Build history of the part. All positions in model axes, mm. Round coordinates to 2 decimals unless told otherwise and drop trailing zeros. Loops run counter-clockwise (first coordinate to the right, second up) from the corner with the lowest first, then second, coordinate; pieces in that order, holes last.
from build123d import *

# Parameters (mm, degrees)
F0_W     = 50.8
F0_H     = 101.6
F0_R     = 7.62
F1_DEPTH = 25.4
F2_R     = 5.08
F3_R     = 3.752901
F4_DEPTH = 25.4


with BuildPart() as f1:
    # F0 (on Front) → F1 (new body)
    with BuildSketch(Plane.XZ):
        Rectangle(F0_W, F0_H)
        with Locations((0, -26.934734)):
            Circle(F0_R, mode=Mode.SUBTRACT)
        with Locations((0, 26.934734)):
            Circle(F0_R, mode=Mode.SUBTRACT)
    extrude(amount=F1_DEPTH)

    # F2
    f2_edges = [f1.edges().sort_by_distance(p)[0] for p in [
        (25.4, -12.7, -50.8),
        (25.4, -12.7, 50.8),
        (-25.4, -12.7, 50.8),
        (-25.4, -12.7, -50.8),
    ]]
    fillet(f2_edges, radius=F2_R)

    # F3 (on face) → F4 (cut)
    with BuildSketch(Plane(origin=(0, 0, 0), x_dir=(-1, 0, 0), z_dir=(0, 1, 0))):
        with Locations((-15.947323, 40.916275)):
            Circle(F3_R)
        with Locations((15.947323, 40.916275)):
            Circle(F3_R)
        with Locations((15.947323, -40.916275)):
            Circle(F3_R)
        with Locations((-15.947323, -40.916275)):
            Circle(F3_R)
    extrude(amount=-F4_DEPTH, mode=Mode.SUBTRACT)


solid = f1.part
(1) Probe line 1 (Z direction, x = 0, y = -19.5); line 2 (X direction, y = -15, z = -40.5); line 3 (Z direction, x = 16, y = -14.5). List the from-to ranges inside material, lowest first.
Responses:
line 1: z = -50.8 to -34.55, -19.31 to 19.31, 34.55 to 50.8
line 2: x = -25.4 to -19.68, -12.22 to 12.22, 19.68 to 25.4
line 3: z = -50.8 to -44.67, -37.16 to 37.16, 44.67 to 50.8
(2) Pin check, flat tip, straight feed: P1, Ø6, axis at x = 15.95, z = 40.92, coming from the +Y side. Stop position of the tip, or through.
Responses:
P1: passes through
(3) Slice it at C-C on y = -12. List the corners of the cut face in (x, z), plus the area to 3 significant figures.
Responses:
outline: (-25.4, -45.72) arc R5.08 ccw to (-20.32, -50.8) - (20.32, -50.8) arc R5.08 ccw to (25.4, -45.72) - (25.4, 45.72) arc R5.08 ccw to (20.32, 50.8) - (-20.32, 50.8) arc R5.08 ccw to (-25.4, 45.72) - close; hole circle Ø7.51 at (-15.95, -40.92); hole circle Ø7.51 at (-15.95, 40.92); hole circle Ø15.24 at (0, -26.93); hole circle Ø15.24 at (0, 26.93); hole circle Ø7.51 at (15.95, -40.92); hole circle Ø7.51 at (15.95, 40.92)
area: 4,600 mm2
(4) Slice it at A-A on x = 0. List the corners of the cut face in (y, z), plus the area to 3 significant figures.
Responses:
outline: (-25.4, -50.8) - (0, -50.8) - (0, -34.55) - (-25.4, -34.55) - close; (-25.4, -19.31) - (0, -19.31) - (0, 19.31) - (-25.4, 19.31) - close; (-25.4, 34.55) - (0, 34.55) - (0, 50.8) - (-25.4, 50.8) - close
area: 1,810 mm2
(5) Slice it at B-B on z = -31.5. List the corners of the cut face in (x, y).
Responses:
outline: (-25.4, -25.4) - (-6.1, -25.4) - (-6.1, 0) - (-25.4, 0) - close; (6.1, -25.4) - (25.4, -25.4) - (25.4, 0) - (6.1, 0) - close
(6) Slice it at D-D on x = -18.5. List the corners of the cut face in (y, z), plus the area to 3 significant figures.
Responses:
outline: (-25.4, -50.8) - (0, -50.8) - (0, -43.67) - (-25.4, -43.67) - close; (-25.4, -38.17) - (0, -38.17) - (0, 38.17) - (-25.4, 38.17) - close; (-25.4, 43.67) - (0, 43.67) - (0, 50.8) - (-25.4, 50.8) - close
area: 2,300 mm2
(7) Pull direction X, two halves, no side cores. Call faces 1 (the face through (-23.951, -12.878, -49.272)), 2 (the face through (0, -13, 50.8)), 3 (the face through (-15.459, -12.522, -37.195)), 4 (the face through (-15.134, -12.522, 37.253)): +X half, -X half, draft (parallel to the pull), parting line (faces both ways), or undercut.
Responses:
face 1: -X half
face 2: draft
face 3: undercut
face 4: undercut
